from build123d import *

# Parameters (mm, degrees)
SKETCH004_W    = 11.5
SKETCH004_H    = 1.25
PAD003_DEPTH   = 3.2
PAD_DEPTH      = 42
PAD_DEPTH_BACK = 1.6
THICKNESS_T    = -0.8
SKETCH002_R    = 1.75
PAD001_DEPTH   = 13
SKETCH003_R    = 3.5
PAD002_DEPTH   = 14
FILLET_R       = 0.6


with BuildPart() as pad003:
    # Sketch004 → Pad003 (new body)
    with BuildSketch(Plane.XZ.offset(46.2)):
        with BuildLine():
            Line((22.5, 29), (37.25, 29))
            ThreePointArc((38.25, 28), (37.957107, 28.707107), (37.25, 29))
            Line((38.25, 28), (38.25, 18))
            ThreePointArc((37.25, 17), (37.957107, 17.292893), (38.25, 18))
            Line((37.25, 17), (22.5, 17))
            ThreePointArc((21.5, 18), (21.792893, 17.292893), (22.5, 17))
            Line((21.5, 18), (21.5, 28))
            ThreePointArc((22.5, 29), (21.792893, 28.707107), (21.5, 28))
        make_face()
        with BuildLine():
            Line((-8.95, 29.8), (-3.75, 29.8))
            ThreePointArc((-2.75, 28.8), (-3.042893, 29.507107), (-3.75, 29.8))
            Line((-2.75, 28.8), (-2.75, 16.5))
            ThreePointArc((-3.75, 15.5), (-3.042893, 15.792893), (-2.75, 16.5))
            Line((-3.75, 15.5), (-8.95, 15.5))
            ThreePointArc((-9.95, 16.5), (-9.657107, 15.792893), (-8.95, 15.5))
            Line((-9.95, 16.5), (-9.95, 28.8))
            ThreePointArc((-8.95, 29.8), (-9.657107, 29.507107), (-9.95, 28.8))
        make_face()
        with BuildLine():
            Line((-37.25, 24.5), (-31.25, 24.5))
            ThreePointArc((-30.25, 23.5), (-30.542893, 24.207107), (-31.25, 24.5))
            Line((-30.25, 23.5), (-30.25, 18))
            ThreePointArc((-31.25, 17), (-30.542893, 17.292893), (-30.25, 18))
            Line((-31.25, 17), (-37.25, 17))
            ThreePointArc((-38.25, 18), (-37.957107, 17.292893), (-37.25, 17))
            Line((-38.25, 18), (-38.25, 23.5))
            ThreePointArc((-37.25, 24.5), (-37.957107, 24.207107), (-38.25, 23.5))
        make_face()
        with Locations((-20.25, 17.625)):
            Rectangle(SKETCH004_W, SKETCH004_H)
        Polygon((2.333401, 7), (2.333401, 11.006851), (3.391764, 12.4), (15.751917, 12.4), (16.833401, 10.855655), (16.833401, 7), align=None)
    extrude(amount=-PAD003_DEPTH)


with BuildPart() as fillet_body:
    # Sketch001 → Pad (new body, two sides)
    with BuildSketch(Plane.XY) as pad_sk:
        with BuildLine():
            Line((-42.65, 45.4), (42.65, 45.4))
            ThreePointArc((48.65, 39.4), (46.892641, 43.642641), (42.65, 45.4))
            Line((48.65, 39.4), (48.65, -39.4))
            ThreePointArc((42.65, -45.4), (46.892641, -43.642641), (48.65, -39.4))
            Line((42.65, -45.4), (-42.65, -45.4))
            ThreePointArc((-48.65, -39.4), (-46.892641, -43.642641), (-42.65, -45.4))
            Line((-48.65, -39.4), (-48.65, 39.4))
            ThreePointArc((-42.65, 45.4), (-46.892641, 43.642641), (-48.65, 39.4))
        make_face()
    extrude(amount=PAD_DEPTH)
    extrude(pad_sk.sketch, amount=-PAD_DEPTH_BACK)

    # Thickness
    thickness_openings = [fillet_body.faces().sort_by_distance(p)[0] for p in [
        (0, 0, 42),
    ]]
    offset(amount=THICKNESS_T, openings=thickness_openings)

    # Sketch002 → Pad001 (new body)
    with BuildSketch(Plane.XY.offset(-0.8)):
        with Locations((-41.25, -36)):
            Circle(SKETCH002_R)
        with Locations((41.25, -36)):
            Circle(SKETCH002_R)
        with Locations((-41.25, 16.5)):
            Circle(SKETCH002_R)
        with Locations((41.25, 36)):
            Circle(SKETCH002_R)
    extrude(amount=PAD001_DEPTH)

    # Sketch003 → Pad002 (new body)
    with BuildSketch(Plane.XY.offset(-0.8)):
        with Locations((41.25, -36)):
            Circle(SKETCH003_R)
        with Locations((41.25, 36)):
            Circle(SKETCH003_R)
        with Locations((-41.25, 16.5)):
            Circle(SKETCH003_R)
        with Locations((-41.25, -36)):
            Circle(SKETCH003_R)
    extrude(amount=PAD002_DEPTH)

    # Cut: cut Pad003
    add(pad003.part, mode=Mode.SUBTRACT)

    # Fillet
    fillet_edges = [fillet_body.edges().sort_by_distance(p)[0] for p in [
        (0, 45.4, -1.6),
        (46.892641, 43.642641, -1.6),
        (48.65, 0, -1.6),
        (46.892641, -43.642641, -1.6),
        (0, -45.4, -1.6),
        (-46.892641, -43.642641, -1.6),
        (-48.65, 0, -1.6),
        (-46.892641, 43.642641, -1.6),
    ]]
    fillet(fillet_edges, radius=FILLET_R)


solid = fillet_body.part
For this review, take the finished solid that the model builds, in its own axes (mm). A direction names the side the tool comes from. Round coordinates to 2 decimals unless told otherwise and drop trailing zeros. Loops run counter-clockwise (first coordinate to the right, second up) from the corner with the lowest first, then second, coordinate; pieces in that order, holes last. Notation, with made-up numbers: (-33, -21) - (4, -21) arc R15 cw to (4, 8) - close; hole circle Ø2 at (4.5, 64). An arc over 180 degrees is marked (long way). Use one line per item in the form item = value.
1) Mouldability with a two-part tool opening along Y and no side actions: class faces 3 (the face through (46.4, 43, 20.9)), 4 (the face through (1, -45.4, 21)), 5 (the face through (-46.846, 43.689, 20.801)), 6 (the face through (1, 1, -0.8)) as pulls with the +Y half, pulls with the -Y half, needs draft (parallel to the pull), parting line crosses it, or undercut.
Solutions:
face_3 = undercut
face_4 = pulls with the -Y half
face_5 = pulls with the +Y half
face_6 = undercut
2) We need section D-D on y = -36. Write out the cut boundary in (x, z), then the cut area to 3 significant figures.
Solutions:
outline = (-48.65, -1) arc R0.6 ccw to (-48.05, -1.6) - (48.05, -1.6) arc R0.6 ccw to (48.65, -1) - (48.65, 42) - (47.85, 42) - (47.85, -0.8) - (44.75, -0.8) - (44.75, 13.2) - (37.75, 13.2) - (37.75, -0.8) - (-37.75, -0.8) - (-37.75, 13.2) - (-44.75, 13.2) - (-44.75, -0.8) - (-47.85, -0.8) - (-47.85, 42) - (-48.65, 42) - close
area = 342 mm2
3) Tool access review of faces 1 (the face through (-46.939, -43.596, 20.801)), 2 (the face through (-47.85, -1, 21)): name each direction out of +Z, -Z, +X, -X, +Y, -Y from which nothing blocks a thin tool from reaching the whole face with its end or side.
Solutions:
face_1 = +Z, -Z, -X, -Y
face_2 = +Z
4) We need section C-C on z = 21. Write out the cut boundary in (x, y).
Solutions:
outline = (-48.65, -39.4) arc R6 ccw to (-42.65, -45.4) - (-38.25, -45.4) - (-38.25, -44.6) - (-42.65, -44.6) arc R5.2 cw to (-47.85, -39.4) - (-47.85, 39.4) arc R5.2 cw to (-42.65, 44.6) - (42.65, 44.6) arc R5.2 cw to (47.85, 39.4) - (47.85, -39.4) arc R5.2 cw to (42.65, -44.6) - (38.25, -44.6) - (38.25, -45.4) - (42.65, -45.4) arc R6 ccw to (48.65, -39.4) - (48.65, 39.4) arc R6 ccw to (42.65, 45.4) - (-42.65, 45.4) arc R6 ccw to (-48.65, 39.4) - close; (-30.25, -45.4) - (-9.95, -45.4) - (-9.95, -44.6) - (-30.25, -44.6) - close; (-2.75, -45.4) - (21.5, -45.4) - (21.5, -44.6) - (-2.75, -44.6) - close
5) We need section A-A on z = 3.5. Write out the cut boundary in (x, y).
Solutions:
outline = (-48.65, -39.4) arc R6 ccw to (-42.65, -45.4) - (42.65, -45.4) arc R6 ccw to (48.65, -39.4) - (48.65, 39.4) arc R6 ccw to (42.65, 45.4) - (-42.65, 45.4) arc R6 ccw to (-48.65, 39.4) - close; circle Ø7 at (-41.25, -36); circle Ø7 at (-41.25, 16.5); circle Ø7 at (41.25, -36); circle Ø7 at (41.25, 36); hole (-47.85, -39.4) arc R5.2 ccw to (-42.65, -44.6) - (42.65, -44.6) arc R5.2 ccw to (47.85, -39.4) - (47.85, 39.4) arc R5.2 ccw to (42.65, 44.6) - (-42.65, 44.6) arc R5.2 ccw to (-47.85, 39.4) - close
6) Clearance check with flat-ended pins moving along their axes: P1, Ø0.9, axis at y = -45, z = 20.5, coming from the -X side; P2, Ø0.6, axis at y = -45, z = 22, coming from the -X side. State where each tip first meets the part, or that it passes through.
Solutions:
P1 = -45.73
P2 = -45.46
7) Wall thickness on probe 1 along Y at (x, z) = (-41, 8.5); probe 2 along X at (y, z) = (-5, 27.5); probe 3 along Y at (x, z) = (6.5, 16): over which ranges is each line inside the solid? List them lowest first.
Solutions:
probe_1 = -45.4 to -44.6, -39.49 to -32.51, 13.01 to 19.99, 44.6 to 45.4
probe_2 = -48.65 to -47.85, 47.85 to 48.65
probe_3 = -45.4 to -44.6, 44.6 to 45.4
8) We need section B-B on x = 13.5. Write out the cut boundary in (y, z), then the cut area to 3 significant figures.
Solutions:
outline = (-45.4, -1) arc R0.6 ccw to (-44.8, -1.6) - (44.8, -1.6) arc R0.6 ccw to (45.4, -1) - (45.4, 42) - (44.6, 42) - (44.6, -0.8) - (-44.6, -0.8) - (-44.6, 7) - (-45.4, 7) - close; (-45.4, 12.4) - (-44.6, 12.4) - (-44.6, 42) - (-45.4, 42) - close
area = 137 mm2
